Autodesk Inventor part; units mm, degrees
ref_plane "YZ Plane" through (0, 0, 0) normal (1, 0, 0) x (0, 1, 0)
ref_plane "XZ Plane" through (0, 0, 0) normal (0, 1, 0) x (-1, 0, 0)
ref_plane "XY Plane" through (0, 0, 0) normal (0, 0, 1) x (1, 0, 0)
sketch "Sketch1" plane through (0, 0, 0) normal (0, 0, 1) x (1, 0, 0)
  line L0 (0, 56.7) -> (0, -56.7) construction
  line L1 (-56.7, 0) -> (56.7, 0) construction
  line L2 (-37.5, 37.5) -> (37.5, 37.5)
  line L3 (37.5, 37.5) -> (37.5, -37.5)
  line L4 (37.5, -37.5) -> (-37.5, -37.5)
  line L5 (-37.5, -37.5) -> (-37.5, 37.5)
  line L6 (-40.5, 40.5) -> (40.5, 40.5)
  line L7 (40.5, 40.5) -> (40.5, -40.5)
  line L8 (40.5, -40.5) -> (-40.5, -40.5)
  line L9 (-40.5, -40.5) -> (-40.5, 40.5)
  point P0 (0, 0)
  dimension "d0" = 75
  dimension "d1" = 75
  dimension "d2" = 3
  dimension "d3" = 3
  dimension "d4" = 3
  dimension "d5" = 3
extrude "Extrusion1" add sketch "Sketch1" along normal blind 150
sketch "Sketch2" plane through (0, 0, 0) normal (0, 0, -1) x (-1, 0, 0)
  line L0 (-40.5, -40.5) -> (40.5, -40.5)
  line L1 (40.5, -40.5) -> (40.5, 40.5)
  line L2 (40.5, 40.5) -> (-40.5, 40.5)
  line L3 (-40.5, 40.5) -> (-40.5, -40.5)
  point P0 (0, 0)
extrude "Extrusion2" add sketch "Sketch2" along normal blind 3
properties part number "Cuvette_75x75x150" material "Glass"
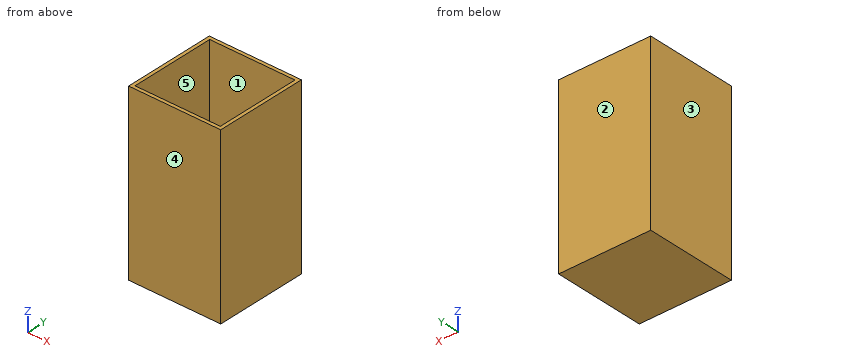
Source: CAD feature listing. Evaluate the final solid. Frame: model axes, mm. Face numbers are marked on the shaded views. A direction names the side the tool comes from. Coordinates: 2 decimals unless noted, no trailing zeros. Loops run counter-clockwise (first coordinate to the right, second up) from the corner with the lowest first, then second, coordinate; pieces in that order, holes last. Notation, with made-up numbers: M -6,42.25 L 13,42.25 A17 ccw 13,57.25 Z; hole C 54,38.5 d10. An arc over 180 degrees is marked long. Put each result on its own line as item: value. Start each with the question number.
1) Cut plane A-A on z = 95. Return the cut outline in (x, y).
2) Contact query for a flat-ended pin moving along its axis: pin 1 Ø1 at (x, y) = (-7.5, -7) entering from +Z. Output: stop coordinate, or through.
3) Ray query, L1, parallel to Y at x = -10, z = 9; L2, parallel to Z at x = -4, y = 5.5. Return the intervals inside material, ascending. Write a range as from..to.
4) Reachability of the marked faces 1 and 2 from +Z, -Z, +X, -X, +Y, -Y: full face, straight path, thin tool, end or side. Return the list, or none.
5) Cut plane B-B on y = -7. Return the cut outline in (x, z), then the cut area to 3 significant figures.
6) Pull-direction query (Y, two-part tool) for the marked faces 3, 4 and 5; classes: pulls with the +Y half, pulls with the -Y half, needs draft (parallel to the pull), parting line crosses it, or undercut.
The answers:
1. outline: M -40.5,-40.5 L 40.5,-40.5 L 40.5,40.5 L -40.5,40.5 Z; hole M -37.5,-37.5 L 37.5,-37.5 L 37.5,37.5 L -37.5,37.5 Z
2. pin 1: stops at z = 0
3. L1: y = -40.5..-37.5, 37.5..40.5
3. L2: z = -3..0
4. face 1: +Z
4. face 2: +Z, -Z, +X, -X, +Y
5. outline: M -40.5,-3 L 40.5,-3 L 40.5,150 L 37.5,150 L 37.5,0 L -37.5,0 L -37.5,150 L -40.5,150 Z
5. area: 1,140 mm²
6. face 3: needs draft
6. face 4: pulls with the -Y half
6. face 5: undercut
